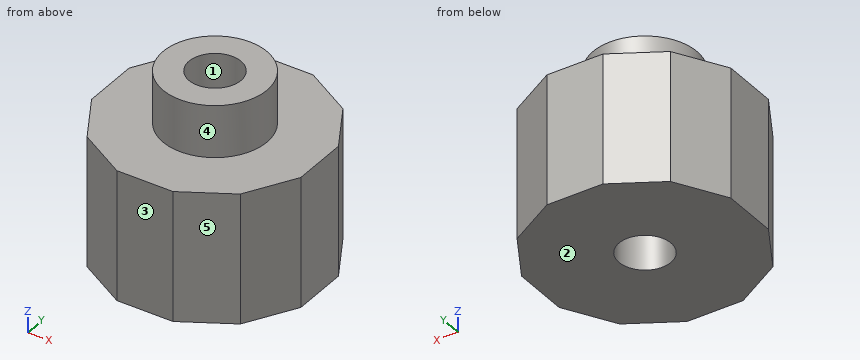
from build123d import *

# Parameters (mm, degrees)
PAD_DEPTH    = 15
SKETCH001_R  = 6
PAD001_DEPTH = 6
SKETCH002_R  = 3
POCKET_DEPTH = 21.001


with BuildPart() as part:
    # Sketch → Pad (new body)
    with BuildSketch(Plane.XY):
        Polygon((8.838835, 8.838835), (3.235238, 12.074073), (-3.235238, 12.074073), (-8.838835, 8.838835), (-12.074073, 3.235238), (-12.074073, -3.235238), (-8.838835, -8.838835), (-3.235238, -12.074073), (3.235238, -12.074073), (8.838835, -8.838835), (12.074073, -3.235238), (12.074073, 3.235238), align=None)
    extrude(amount=PAD_DEPTH)

    # Sketch001 (on Face14 of Pad) → Pad001 (join)
    with BuildSketch(Plane.XY.offset(15)):
        Circle(SKETCH001_R)
    extrude(amount=PAD001_DEPTH)

    # Sketch002 (on Face16 of Pad001) → Pocket (cut, through all)
    with BuildSketch(Plane.XY.offset(21)):
        Circle(SKETCH002_R)
    extrude(amount=-POCKET_DEPTH, mode=Mode.SUBTRACT)


solid = part.part
The model under review builds one solid part; all positions refer to its coordinate system, in mm. Face numbers are marked on the shaded views. A direction names the side the tool comes from. Round coordinates to 2 decimals unless told otherwise and drop trailing zeros. Write each loop counter-clockwise with the first axis right and the second up, starting at its lowest first coordinate (ties: lowest second). Pieces come first, ordered by that corner, then holes. Notation, with made-up numbers: M 29,-10 L 82,-10 A26 ccw 82,6 Z; hole C -22,-34 d8. An arc over 180 degrees is marked long. Use a Markdown table: item, result. Add a question column.
Q1. We need section D-D, the plane x = 4.5. State the section outline as (y, z) points, plus the area to 3 significant figures.
Q2. Insertion check: pin 1 (5 mm diameter, centred on y = 6, z = 7, fed in from +X); pin 2 (5 mm diameter, centred on y = 8, z = 4.5, fed in from -X); pin 3 (2 mm diameter, centred on x = 9, z = 5.5, fed in from +Y). Each pin has a flat end and moves straight along its axis. Give the tip position at first contact, or say it passes through.
Q3. We need section A-A, the plane x = 0. State the section outline as (y, z) points, plus the area to 3 significant figures.
Q4. The part is to be moulded in two halves that separate along Y. For the marked faces 1, 2 and 3, say which applies: pulls with the +Y half, pulls with the -Y half, needs draft (parallel to the pull), parting line crosses it, or undercut.
Q5. To check wall thickness, follow line 1 (Y direction, x = 0, z = 11.25); line 2 (Z direction, x = 2.75, y = 10.25); line 3 (Y direction, x = -2, z = 14.25). State the ranges of each line that lie inside material, in increasing order.
Q6. Machinability: for the marked faces 4 and 5, which of the approach directions +Z, -Z, +X, -X, +Y, -Y give a long, thin tool a straight path to every point of the face, cutting with its end or side? Answer none if there is none.
Q7. We need section C-C, the plane z = 11.75. State the section outline as (x, y) points, plus the area to 3 significant figures.
Findings below:
| question | item | result |
|---|---|---|
| 1 | outline | M -11.34,0 L 11.34,0 L 11.34,15 L 3.97,15 L 3.97,21 L -3.97,21 L -3.97,15 L -11.34,15 Z |
| 1 | area | 388 mm² |
| 2 | pin 1 | stops at x = 11.92 |
| 2 | pin 2 | stops at x = -10.77 |
| 2 | pin 3 | stops at y = 9.32 |
| 3 | outline | M -12.07,0 L -3,0 L -3,21 L -6,21 L -6,15 L -12.07,15 Z; M 3,0 L 12.07,0 L 12.07,15 L 6,15 L 6,21 L 3,21 Z |
| 3 | area | 308 mm² |
| 4 | face 1 | undercut |
| 4 | face 2 | needs draft |
| 4 | face 3 | pulls with the -Y half |
| 5 | line 1 | y = -12.07 to -3, 3 to 12.07 |
| 5 | line 2 | z = 0 to 15 |
| 5 | line 3 | y = -12.07 to -2.24, 2.24 to 12.07 |
| 6 | face 4 | +Z |
| 6 | face 5 | +Z, -Z, +X, -Y |
| 7 | outline | M -12.07,-3.24 L -8.84,-8.84 L -3.24,-12.07 L 3.24,-12.07 L 8.84,-8.84 L 12.07,-3.24 L 12.07,3.24 L 8.84,8.84 L 3.24,12.07 L -3.24,12.07 L -8.84,8.84 L -12.07,3.24 Z; hole C 0,0 d6 |
| 7 | area | 440 mm² |
